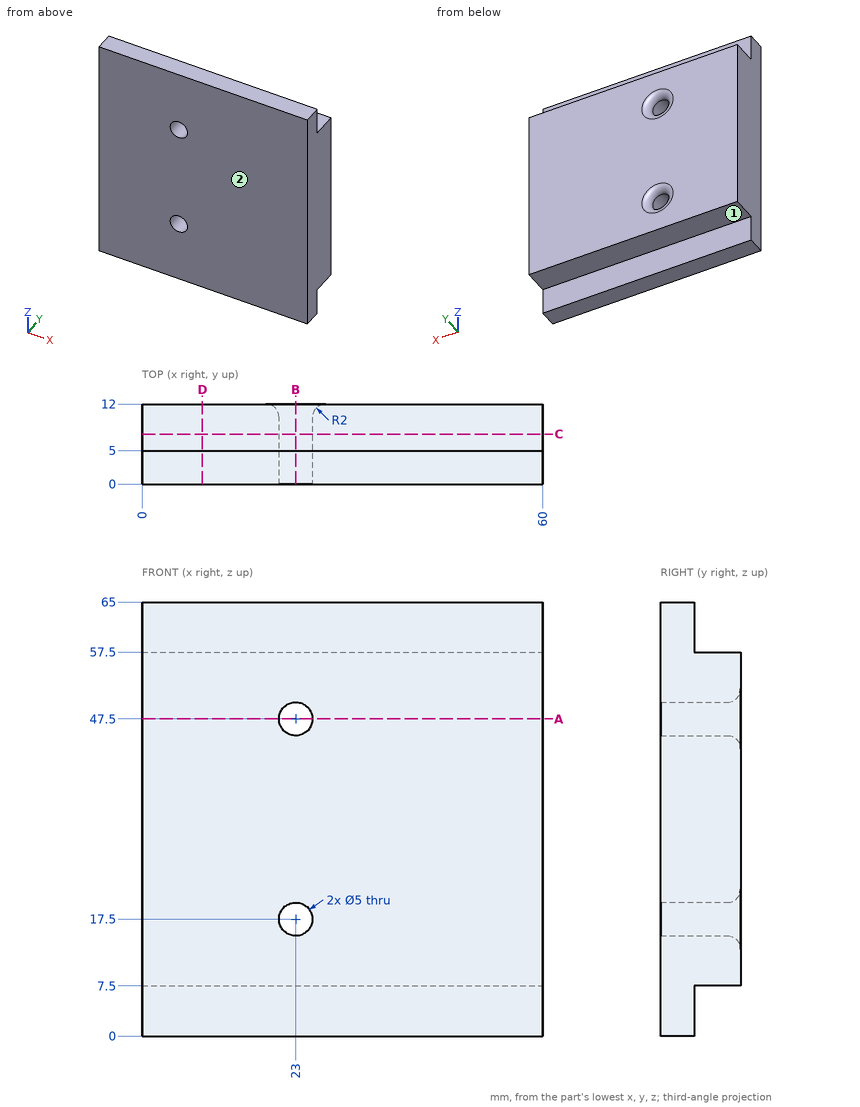
Job drawing, mm, ordinate dimensions from the low corner. One solid piece. A direction names the side the tool comes from. Give positions to 0.01 mm unless a question says otherwise; leave off trailing zeros. Write each loop counter-clockwise with the first axis right and the second up, starting at its lowest first coordinate (ties: lowest second). Pieces come first, ordered by that corner, then holes. Notation, with made-up numbers: M -30.5,31.25 L 18.5,31.25 A18 cw 18.5,62.25 Z; hole C -26,0 d4. An arc over 180 degrees is marked long. Put each result on its own line as item: value. Start each with the question number.
(1) Which spindle directions (+Z, -Z, +X, -X, +Y, -Y) get a long thin tool onto all of the face, cutting with end or side? Do the marked faces 1 and 2. Say none if no direction does.
(2) Band-saw the part on B-B, the plane x = 23. Write the cut outline in (y, z).
(3) Band-saw the part on C-C, the plane y = 7.5. Write the cut outline in (x, z), and give its area (3 significant figures).
(4) Band-saw the part on D-D, the plane x = 9. Write the cut outline in (y, z), and give its area (3 significant figures).
(5) Band-saw the part on A-A, the plane z = 47.5. Write the cut outline in (x, y), and give its area (3 significant figures).
(6) Probe L1, parallel to Z at x = 23, y = 7; L2, parallel to X at y = 3, z = 47.5; L3, parallel to Z at x = 23, y = 3.5. List the from-to ranges inside material, lowest first.
(7) Flat gauge pins, fed straight in: pin 1 Ø6 at (x, z) = (16.5, 3) entering from +Y; pin 2 Ø3.5 at (x, y) = (21.5, 10) entering from +Z; pin 3 Ø8 at (x, z) = (23, 47.5) entering from +Y. Where does each tip first touch, or does it go through?
Response values:
1. face 1: -Z, +X, -X, +Y
1. face 2: +Z, -Z, +X, -X, -Y
2. outline: M 0,0 L 5,0 L 5,7.5 L 12,7.5 L 12,13 A2 ccw 10,15 L 0,15 Z; M 0,20 L 10,20 A2 ccw 12,22 L 12,43 A2 ccw 10,45 L 0,45 Z; M 0,50 L 10,50 A2 ccw 12,52 L 12,57.5 L 5,57.5 L 5,65 L 0,65 Z
3. outline: M 0,7.5 L 60,7.5 L 60,57.5 L 0,57.5 Z; hole C 23,17.5 d5; hole C 23,47.5 d5
3. area: 2,960 mm2
4. outline: M 0,0 L 5,0 L 5,7.5 L 12,7.5 L 12,57.5 L 5,57.5 L 5,65 L 0,65 Z
4. area: 675 mm2
5. outline: M 0,0 L 20.5,0 L 20.5,10 A2 ccw 18.5,12 L 0,12 Z; M 25.5,0 L 60,0 L 60,12 L 27.5,12 A2 ccw 25.5,10 Z
5. area: 658 mm2
6. L1: z = 7.5 to 15, 20 to 45, 50 to 57.5
6. L2: x = 0 to 20.5, 25.5 to 60
6. L3: z = 0 to 15, 20 to 45, 50 to 65
7. pin 1: stops at y = 5
7. pin 2: stops at z = 57.5
7. pin 3: stops at y = 11.94
